Could you check a few things on this drawing? It's one solid part, dimensions in mm from its lowest x, y, z. A direction names the side the tool comes from. Give positions to 0.01 mm unless a question says otherwise; leave off trailing zeros. Order: outer loops, then holes, each group sorted by start corner. A loop starts at its lowest first (then second) coordinate and runs counter-clockwise, first axis right, second up.
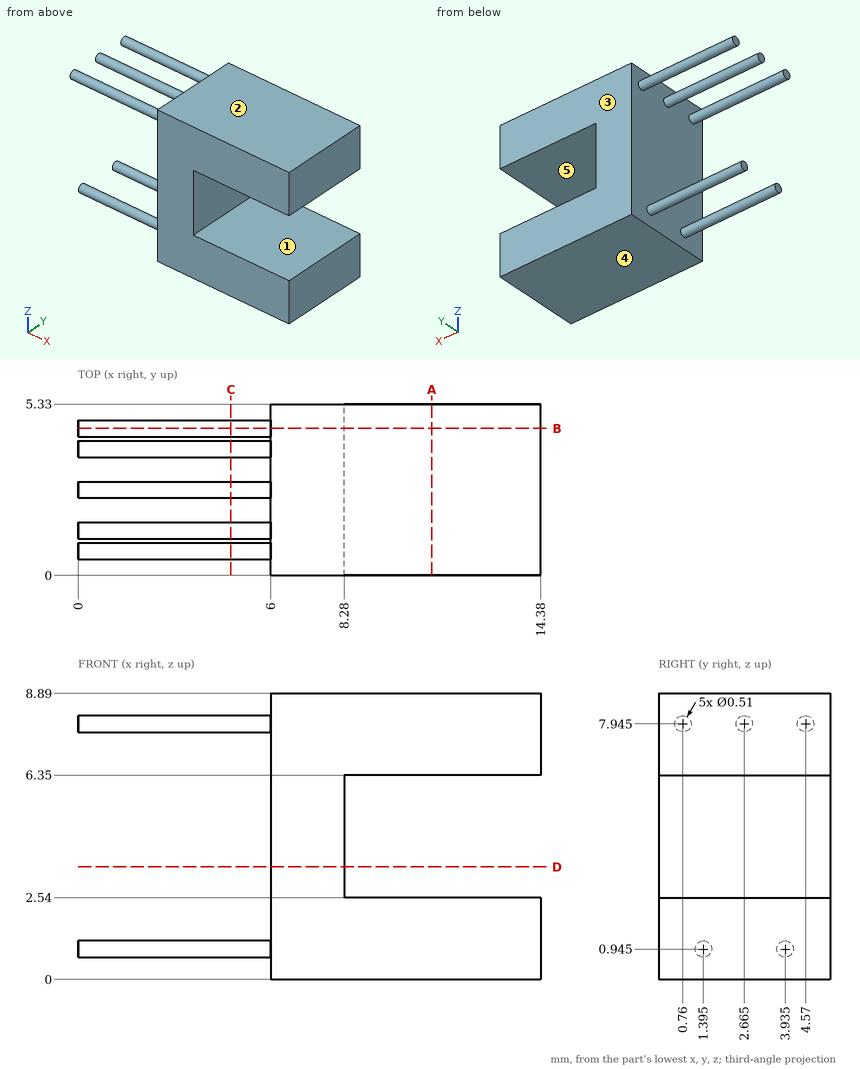
Item 1: Imagine slicing it at D-D on z = 3.5. List the corners of the cut face in (x, y) for me, then the cut area to 3 significant figures.
Findings:
outline: (6, 0) - (8.28, 0) - (8.28, 5.33) - (6, 5.33) - close
area: 12.2 mm2
Item 2: For the marked faces 1 and 2, which set-ups out of +Z, -Z, +X, -X, +Y, -Y let a thin tool reach every point of the face, with its end or its side?
Findings:
face 1: +X, +Y, -Y
face 2: +Z, +X, -X, +Y, -Y
Item 3: We'd pull the mould along Z, two halves only. Please class the marked faces 3, 4 and 5: +Z half, -Z half, draft (parallel to the pull), parting line (faces both ways), or undercut.
Findings:
face 3: draft
face 4: -Z half
face 5: undercut
Item 4: For pin 1 (1.9 mm diameter, centred on y = 2, z = 4.5, fed in from +X), with a flat end and sliding along its axis, tell me the tip position at first contact or that it passes through.
Findings:
pin 1: stops at x = 8.28
Item 5: Imagine slicing it at B-B on y = 4.57. List the corners of the cut face in (x, z) for me.
Findings:
outline: (0, 7.69) - (6, 7.69) - (6, 0) - (14.38, 0) - (14.38, 2.54) - (8.28, 2.54) - (8.28, 6.35) - (14.38, 6.35) - (14.38, 8.89) - (6, 8.89) - (6, 8.2) - (0, 8.2) - close
Item 6: Please list where these lines run through material, in increasing order: line 1 along Z through (x, y) = (8.75, 2.9); line 2 along X through (y, z) = (1.65, 7.25); line 3 along X through (y, z) = (5.05, 4.75).
Findings:
line 1: z = 0 to 2.54, 6.35 to 8.89
line 2: x = 6 to 14.38
line 3: x = 6 to 8.28
Item 7: Imagine slicing it at A-A on x = 11. List the corners of the cut face in (y, z) for me.
Findings:
outline: (0, 0) - (5.33, 0) - (5.33, 2.54) - (0, 2.54) - close; (0, 6.35) - (5.33, 6.35) - (5.33, 8.89) - (0, 8.89) - close
Item 8: Imagine slicing it at C-C on x = 4.75. List the corners of the cut face in (y, z) for me (3 decimals), then the cut area to 3 significant figures.
Findings:
outline: circle Ø0.51 at (0.76, 7.945); circle Ø0.51 at (1.395, 0.945); circle Ø0.51 at (2.665, 7.945); circle Ø0.51 at (3.935, 0.945); circle Ø0.51 at (4.57, 7.945)
area: 1.02 mm2
